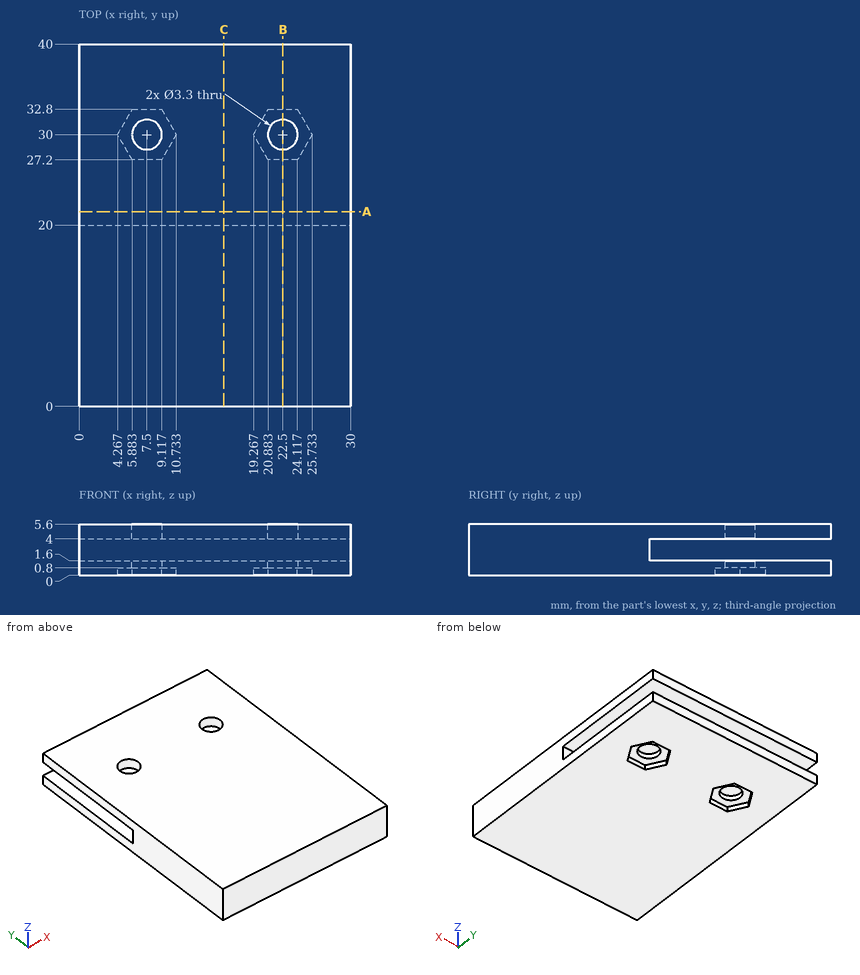
Source: three-view drawing plus pictorial views. Frame: mm from the lowest corner of the part. Coordinates: 2 decimals unless noted, no trailing zeros. Write each loop counter-clockwise with the first axis right and the second up, starting at its lowest first coordinate (ties: lowest second). Pieces come first, ordered by that corner, then holes. Notation, with made-up numbers: (14, 80.25) - (39, 80.25) arc R20 cw to (39, 86.25) - close; hole circle Ø8 at (-21, 83.25). An arc over 180 degrees is marked (long way). Return JSON: item names as keys, results as strings.
Item 1: Section query B-B (x = 22.5). Output: boundary loops of the cut face in (y, z).
Completed:
{"outline": "(0, 0) - (27.2, 0) - (27.2, 0.8) - (28.35, 0.8) - (28.35, 1.6) - (20, 1.6) - (20, 4) - (28.35, 4) - (28.35, 5.6) - (0, 5.6) - close; (31.65, 0.8) - (32.8, 0.8) - (32.8, 0) - (40, 0) - (40, 1.6) - (31.65, 1.6) - close; (31.65, 4) - (40, 4) - (40, 5.6) - (31.65, 5.6) - close"}
Item 2: Section query A-A (y = 21.5). Output: boundary loops of the cut face in (x, z).
Completed:
{"outline": "(0, 0) - (30, 0) - (30, 1.6) - (0, 1.6) - close; (0, 4) - (30, 4) - (30, 5.6) - (0, 5.6) - close"}
Item 3: Pin query (flat end, axial travel): pin 1 Ø5.5 at (x, y) = (7.5, 30) entering from -Z; pin 2 Ø4 at (x, y) = (26.5, 18.5) entering from -Z. Return the tip coordinate at first contact, or that it passes through.
Completed:
{"pin 1": "stops at z = 0.8", "pin 2": "stops at z = 0"}
Item 4: Section query C-C (x = 16). Output: boundary loops of the cut face in (y, z), and give its area (3 significant figures).
Completed:
{"outline": "(0, 0) - (40, 0) - (40, 1.6) - (20, 1.6) - (20, 4) - (40, 4) - (40, 5.6) - (0, 5.6) - close", "area": "176 mm2"}
Item 5: Line query: L1, parallel to Z at x = 20.5, y = 33; L2, parallel to Y at x = 21, z = 0.7; L3, parallel to Y at x = 7.5, z = 5.2. Output: solid intervals per line, ascending.
Completed:
{"L1": "z = 0 to 1.6, 4 to 5.6", "L2": "y = 0 to 27.2, 32.8 to 40", "L3": "y = 0 to 28.35, 31.65 to 40"}
